```python
from build123d import *

# Parameters (mm, degrees)
CROQUIS6_R            = 2.25
CORTAR_EXTRUIR3_DEPTH = 7
CROQUIS7_R            = 3.75
CORTAR_EXTRUIR4_DEPTH = 4.5


with BuildPart() as part:
    # Croquis5 → Revolución1 (revolve)
    with BuildSketch(Plane(origin=(0, 0, 0), x_dir=(0, 0, -1), z_dir=(1, 0, 0))):
        Polygon((0, 6), (-57, 6), (-57, 10.5), (-6, 10.5), (-6, 21), (0, 21), align=None)
    revolve(axis=Axis((0, 0, 0), (0, 0, 1)))

    # Croquis6 → Cortar-Extruir3 (cut, through all)
    with BuildSketch(Plane.XY.offset(6)):
        with Locations((0, 16)):
            Circle(CROQUIS6_R)
        with Locations((16, 0)):
            Circle(CROQUIS6_R)
        with Locations((0, -16)):
            Circle(CROQUIS6_R)
        with Locations((-16, 0)):
            Circle(CROQUIS6_R)
    extrude(amount=-CORTAR_EXTRUIR3_DEPTH, mode=Mode.SUBTRACT)

    # Croquis7 → Cortar-Extruir4 (cut)
    with BuildSketch(Plane(origin=(0, 0, 0), x_dir=(-1, 0, 0), z_dir=(0, 0, -1))):
        with Locations((0, 16)):
            Circle(CROQUIS7_R)
        with Locations((16, 0)):
            Circle(CROQUIS7_R)
        with Locations((0, -16)):
            Circle(CROQUIS7_R)
        with Locations((-16, 0)):
            Circle(CROQUIS7_R)
    extrude(amount=-CORTAR_EXTRUIR4_DEPTH, mode=Mode.SUBTRACT)


solid = part.part
```
Can you work these out from the model? Positions are in its coordinate system, mm. A direction names the side the tool comes from. Coordinates: 2 decimals unless noted, no trailing zeros. Order: outer loops, then holes, each group sorted by start corner. A loop starts at its lowest first (then second) coordinate and runs counter-clockwise, first axis right, second up.
1. For faces 1 (the face through (-10, -4, 6)), 2 (the face through (-18, -2, 4.5)), 3 (the face through (-0.488, 13.804, 5.26)), which set-ups out of +Z, -Z, +X, -X, +Y, -Y let a thin tool reach every point of the face, with its end or its side?
2. If we section it at C-C (y = 17.5): Please give me the cut outline in (x, z), then the cut area to 3 significant figures.
3. Thinking about a two-plate mould opening in Y: for faces 4 (the face through (5, -5, 57)), 5 (the face through (-13.854, 0.676, 5.26)), 6 (the face through (-3.2, 10, 31.1)), which applies, +Y half, -Y half, draft (parallel to the pull), parting line (faces both ways), or undercut?
4. If we section it at D-D (z = 45.5): Please give me the cut outline in (x, y), then the cut area to 3 significant figures.
5. If we section it at A-A (y = 0): Please give me the cut outline in (x, z).
6. I'm going to push flat-ended pins straight in: pin 1 (4 mm diameter, centred on x = 16.5, y = 0.5, fed in from -Z); pin 2 (1.5 mm diameter, centred on y = -7, z = 33.5, fed in from -X); pin 3 (1 mm diameter, centred on y = 2, z = 44.5, fed in from +X). Where does each tip first touch, or does it pass through?
7. If we section it at B-B (x = 16): Please give me the cut outline in (y, z), then the cut area to 3 significant figures.
8. I need wall thicknesses on line 1 (Y direction, x = 0, z = 2); line 2 (Z direction, x = 11.5, y = 5.5); line 3 (X direction, y = -4, z = 23). Which ranges of each line are inside material? Lowest first, please.
Entries:
1. face 1: +Z
1. face 2: -Z
1. face 3: +Z, -Z
2. outline: (-11.61, 0) - (-3.44, 0) - (-3.44, 4.5) - (-1.68, 4.5) - (-1.68, 6) - (-11.61, 6) - close; (1.68, 4.5) - (3.44, 4.5) - (3.44, 0) - (11.61, 0) - (11.61, 6) - (1.68, 6) - close
2. area: 103 mm2
3. face 4: draft
3. face 5: undercut
3. face 6: parting line
4. outline: circle Ø21 at (0, 0); hole circle Ø12 at (0, 0)
4. area: 233 mm2
5. outline: (-21, 0) - (-19.75, 0) - (-19.75, 4.5) - (-18.25, 4.5) - (-18.25, 6) - (-21, 6) - close; (-13.75, 4.5) - (-12.25, 4.5) - (-12.25, 0) - (-6, 0) - (-6, 57) - (-10.5, 57) - (-10.5, 6) - (-13.75, 6) - close; (6, 0) - (12.25, 0) - (12.25, 4.5) - (13.75, 4.5) - (13.75, 6) - (10.5, 6) - (10.5, 57) - (6, 57) - close; (18.25, 4.5) - (19.75, 4.5) - (19.75, 0) - (21, 0) - (21, 6) - (18.25, 6) - close
6. pin 1: stops at z = 4.5
6. pin 2: stops at x = -8.44
6. pin 3: stops at x = 10.39
7. outline: (-13.6, 0) - (-3.75, 0) - (-3.75, 4.5) - (-2.25, 4.5) - (-2.25, 6) - (-13.6, 6) - close; (2.25, 4.5) - (3.75, 4.5) - (3.75, 0) - (13.6, 0) - (13.6, 6) - (2.25, 6) - close
7. area: 123 mm2
8. line 1: y = -21 to -19.75, -12.25 to -6, 6 to 12.25, 19.75 to 21
8. line 2: z = 0 to 6
8. line 3: x = -9.71 to -4.47, 4.47 to 9.71
